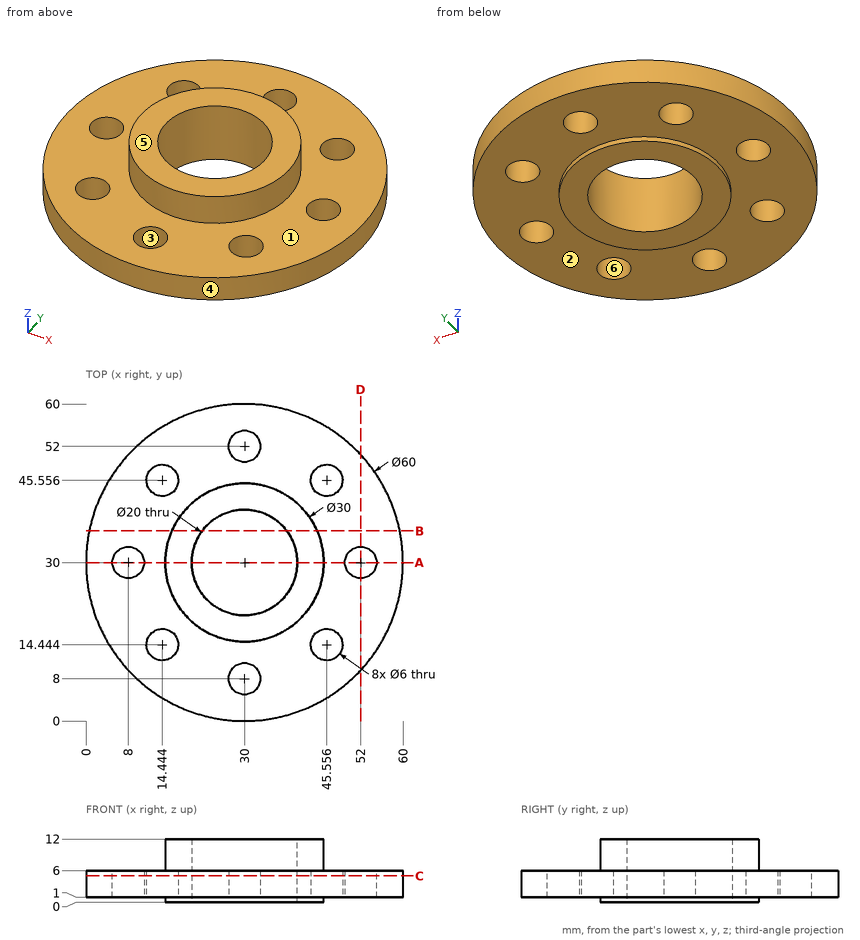
Geometry check sheet. Reference: drawing and pictorial views, mm from the part's lowest x, y, z. A direction names the side the tool comes from. Round coordinates to 2 decimals unless told otherwise and drop trailing zeros. Loops run counter-clockwise (first coordinate to the right, second up) from the corner with the lowest first, then second, coordinate; pieces in that order, holes last. Notation, with made-up numbers: (21, 87) -> (73, 87) arc R19 ccw to (73, 107) -> close; hole circle Ø7 at (-33.75, 72). An arc over 180 degrees is marked (long way). Answer as a JSON object with one key per item and string values.
Q1. Section check D-D (x = 52). Record the boundary of the cut face in (y, z), then the cut area to 3 significant figures.
Data:
{"outline": "(9.6, 1) -> (27, 1) -> (27, 6) -> (9.6, 6) -> close; (33, 1) -> (50.4, 1) -> (50.4, 6) -> (33, 6) -> close", "area": "174 mm2"}
Q2. Section check B-B (y = 36). Record the boundary of the cut face in (x, z).
Data:
{"outline": "(0.61, 1) -> (16.25, 1) -> (16.25, 0) -> (22, 0) -> (22, 12) -> (16.25, 12) -> (16.25, 6) -> (0.61, 6) -> close; (38, 0) -> (43.75, 0) -> (43.75, 1) -> (59.39, 1) -> (59.39, 6) -> (43.75, 6) -> (43.75, 12) -> (38, 12) -> close"}
Q3. Draft check along Y on the marked faces 4, 5 and 6. Enter one of: pulls with the +Y half, pulls with the -Y half, needs draft (parallel to the pull), parting line crosses it, or undercut.
Data:
{"face 4": "parting line crosses it", "face 5": "needs draft", "face 6": "undercut"}
Q4. Section check C-C (z = 5). State how many separate pieces and enclosed holes the cut face has, then the cut area to 3 significant figures.
Data:
{"separate pieces": "1", "enclosed holes": "9", "area": "2,290 mm2"}
Q5. Access from +Z, -Z, +X, -X, +Y, -Y to the whole of each face (thin tool, end or side, straight path). Record for the marked faces 1, 2 and 3.
Data:
{"face 1": "+Z", "face 2": "-Z", "face 3": "+Z, -Z"}
Q6. Scan lines: line 1 (Z direction, x = 8.5, y = 37); line 2 (X direction, y = 21, z = 3.5) (1 decimal); line 3 (Y direction, x = 52, z = 3.75) (1 decimal). Record each from-to range of solid material in increasing order. Write a range as from..to.
Data:
{"line 1": "z = 1..6", "line 2": "x = 1.4..25.6, 34.4..58.6", "line 3": "y = 9.6..27, 33..50.4"}
Q7. Section check A-A (y = 30). Record the boundary of the cut face in (x, z), then the cut area to 3 significant figures.
Data:
{"outline": "(0, 1) -> (5, 1) -> (5, 6) -> (0, 6) -> close; (11, 1) -> (15, 1) -> (15, 0) -> (20, 0) -> (20, 12) -> (15, 12) -> (15, 6) -> (11, 6) -> close; (40, 0) -> (45, 0) -> (45, 1) -> (49, 1) -> (49, 6) -> (45, 6) -> (45, 12) -> (40, 12) -> close; (55, 1) -> (60, 1) -> (60, 6) -> (55, 6) -> close", "area": "210 mm2"}
Q8. Go/stop test with flat-tipped pins: P1, Ø5, axis at x = 14.44, y = 45.56, coming from the -Z side; P2, Ø6, axis at y = 23, z = 7.5, coming from the +X side (1 decimal); P3, Ø8, axis at x = 14.44, y = 14.44, coming from the +Z side. Record where each tip stops, or that it passes through.
Data:
{"P1": "passes through", "P2": "stops at x = 59.7", "P3": "stops at z = 6"}
